The model under review builds one solid part; all positions refer to its coordinate system, in mm. Round coordinates to 2 decimals unless told otherwise and drop trailing zeros. Loops run counter-clockwise (first coordinate to the right, second up) from the corner with the lowest first, then second, coordinate; pieces in that order, holes last. Notation, with made-up numbers: M 87.5,44.5 L 96.5,44.5 A20 ccw 96.5,53.5 Z; hole C 27,58.5 d9. An arc over 180 degrees is marked long. Answer as a JSON object with one key per item and string values. Group by question number.
Item 1: Consider section B-B (y = 1.2). Give the boundary of the cut face in (x, z), and give its area (3 significant figures).
Item 2: To check wall thickness, follow line 1 (X direction, y = 0.9, z = 72); line 2 (Z direction, x = -69, y = 0.5); line 3 (X direction, y = 0.6, z = -4). State the ranges of each line that lie inside material, in increasing order.
Item 3: Insertion check: P1, Ø1.5, axis at x = 17.5, z = 61, coming from the -Y side. The pin has a flat end and moves straight along its axis. Give the tip position at first contact, or say it passes through.
Item 4: Consider section A-A (x = -103.5). Give the boundary of the cut face in (y, z).
Item 5: Consider section C-C (z = 6.5). Give the boundary of the cut face in (x, y).
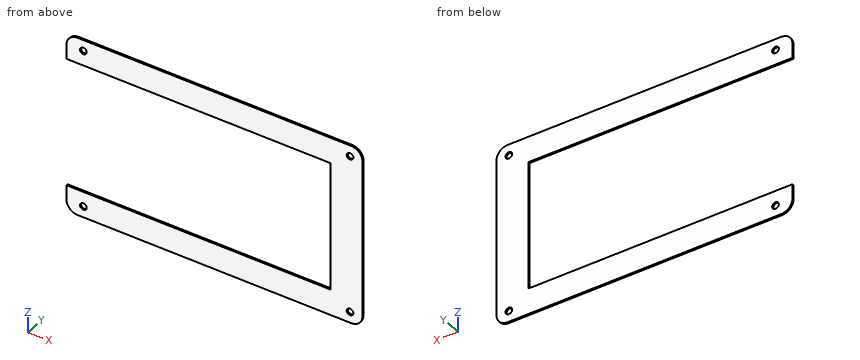
```python
from build123d import *

# Parameters (mm, degrees)
SKETCH1_R          = 3
BASE_FLANGE1_DEPTH = 1.5


# Sheet-metal steps are written as plain solids
with BuildPart() as part:
    # Sketch1 → Base-Flange1 (new body)
    with BuildSketch(Plane(origin=(0, 0, 0), x_dir=(1, 0, 0), z_dir=(0, 1, 0))):
        with BuildLine():
            Line((-127.207269821, 58.5), (-127.207269821, 72))
            ThreePointArc((-127.207269821, 72), (-124.278337633, 79.071067812), (-117.207269821, 82))
            Line((-117.207269821, 82), (126.792730179, 82))
            ThreePointArc((126.792730179, 82), (133.863797991, 79.071067812), (136.792730179, 72))
            Line((136.792730179, 72), (136.792730179, -72))
            ThreePointArc((136.792730179, -72), (133.863797991, -79.071067812), (126.792730179, -82))
            Line((126.792730179, -82), (-117.207269821, -82))
            ThreePointArc((-117.207269821, -82), (-124.278337633, -79.071067812), (-127.207269821, -72))
            Line((-127.207269821, -72), (-127.207269821, -58.5))
            Line((-127.207269821, -58.5), (108.292730179, -58.5))
            Line((108.292730179, -58.5), (108.292730179, 58.5))
            Line((108.292730179, 58.5), (-127.207269821, 58.5))
        make_face()
        with Locations(Location((125.792730179, 72, 0), (0, 0, 270))):
            Circle(SKETCH1_R, mode=Mode.SUBTRACT)
        with Locations(Location((-112.207269821, 72, 0), (0, 0, 270))):
            Circle(SKETCH1_R, mode=Mode.SUBTRACT)
        with Locations(Location((-112.207269821, -72, 0), (0, 0, 270))):
            Circle(SKETCH1_R, mode=Mode.SUBTRACT)
        with Locations(Location((125.792730179, -72, 0), (0, 0, 270))):
            Circle(SKETCH1_R, mode=Mode.SUBTRACT)
    extrude(amount=BASE_FLANGE1_DEPTH)


solid = part.part
```
Geometry results:
{
 "1": {"outline": "M -127.21,-72 A10 ccw -117.21,-82 L 126.79,-82 A10 ccw 136.79,-72 L 136.79,72 A10 ccw 126.79,82 L -117.21,82 A10 ccw -127.21,72 L -127.21,58.5 L 108.29,58.5 L 108.29,-58.5 L -127.21,-58.5 Z; hole C -112.21,-72 d6; hole C -112.21,72 d6; hole C 125.79,-72 d6; hole C 125.79,72 d6", "area": "15,500 mm^2"},
 "2": {"line 1": "x = -127.21 to -115.21, -109.21 to 122.79, 128.79 to 136.79", "line 2": "z = -82 to -58.5, 58.5 to 82", "line 3": "x = 108.29 to 136.79"},
 "3": {"P1": "stops at y = 0"},
 "4": {"outline": "M 0,-82 L 1.5,-82 L 1.5,-58.5 L 0,-58.5 Z; M 0,58.5 L 1.5,58.5 L 1.5,82 L 0,82 Z"},
 "5": {"outline": "M 108.29,0 L 136.79,0 L 136.79,1.5 L 108.29,1.5 Z"}
}
